Could you check a few things on this model? Use its own coordinates, in mm. A direction names the side the tool comes from. Give positions to 0.01 mm unless a question says otherwise; leave off trailing zeros. Loops run counter-clockwise (first coordinate to the right, second up) from the corner with the lowest first, then second, coordinate; pieces in that order, holes last. Notation, with made-up numbers: (-31, -33.5) -> (17, -33.5) arc R23 ccw to (17, -9.5) -> close; hole circle Ø5 at (-8.5, 16.25). An arc over 180 degrees is marked (long way). Put each result on its own line as item: value.
Autodesk Inventor part; units mm, degrees
ref_plane "bnt_nut_1_XY" through (0, 0, 0) normal (1, 0, 0) x (0, 0, -1)
ref_plane "bnt_nut_1_YZ" through (0, 0, 0) normal (0, 0, -1) x (0, 1, 0)
ref_plane "bnt_nut_1_ZX" through (0, 0, 0) normal (0, 1, 0) x (1, 0, 0)
sketch "Sketch_1" plane through (0, 0, 0) normal (1, 0, 0) x (0, 1, 0)
  line L0 (16.56, 24) -> (9, 24)
  line L1 (9, 24) -> (7.56, 22.56)
  line L2 (7.56, 22.56) -> (-13.14, 22.56)
  line L3 (-13.14, 22.56) -> (-13.14, 18)
  arc A0 (-13.14, 18) -> (-23.4, 9.44) centre (-13.3579, 7.8323) ccw
  line L4 (-23.4, 9.44) -> (-23.4, -9.44)
  arc A1 (-23.4, -9.44) -> (-13.14, -18) centre (-13.3579, -7.8323) ccw
  line L5 (-13.14, -18) -> (-13.14, -22.56)
  line L6 (-13.14, -22.56) -> (7.56, -22.56)
  line L7 (7.56, -22.56) -> (9, -24)
  line L8 (9, -24) -> (16.56, -24)
  line L9 (16.56, -24) -> (18, -22.56)
  line L10 (18, -22.56) -> (18, -9.44)
  line L11 (18, -9.44) -> (16.56, -8)
  line L12 (16.56, -8) -> (16.56, 8)
  line L13 (16.56, 8) -> (18, 9.44)
  line L14 (18, 9.44) -> (18, 22.56)
  line L15 (18, 22.56) -> (16.56, 24)
  circle A2 centre (0, 0) radius 10
extrude "Extrusion1" add sketch "Sketch_1" along normal blind 58
sketch "Sketch_2" plane through (29, 0, 0) normal (0.682, 0, 0.7314) x (0.7314, 0, -0.682)
  line L0 (-29, -24.55) -> (-4.4539, -24.55)
  arc A0 (-4.4539, -24.55) -> (4.4539, -24.55) centre (0, -23.4) ccw
  line L1 (4.4539, -24.55) -> (29, -24.55)
  line L2 (29, -24.55) -> (29, -23.4)
  line L3 (29, -23.4) -> (-29, -23.4)
  line L4 (-29, -23.4) -> (-29, -24.55)
extrude "Extrusion2" add sketch "Sketch_2" along normal mid plane 58
sketch "Sketch_3" plane through (0, -23.4, 0) normal (0, 1, 0) x (1, 0, 0)
  line L0 (-29, -58) -> (87, -58)
  line L1 (87, -58) -> (87, 58)
  line L2 (87, 58) -> (-29, 58)
  line L3 (-29, 58) -> (-29, -58)
  line L4 (9.6667, -9.44) -> (48.3333, -9.44)
  line L5 (48.3333, -9.44) -> (48.3333, 9.44)
  line L6 (48.3333, 9.44) -> (9.6667, 9.44)
  line L7 (9.6667, 9.44) -> (9.6667, -9.44)
extrude "Extrusion3" cut sketch "Sketch_3" against normal blind 4.6
sketch "Sketch_4" plane through (0, 0, 0) normal (0, 0, 1) x (1, 0, 0)
  line L0 (13.4367, -26.15) -> (13.4367, -24.55)
  line L1 (13.4367, -24.55) -> (15.4367, -24.55)
  line L2 (15.4367, -24.55) -> (15.4367, -25.75)
  arc A0 (15.0367, -26.15) -> (15.4367, -25.75) centre (15.0367, -25.75) ccw
  line L3 (15.0367, -26.15) -> (13.4367, -26.15)
  line L4 (13.4367, -26.15) -> (13.4367, -24.55)
revolve "Revolution1" add sketch "Sketch_4" angle 360 about axis through (13.4367, -26.15, 0) along (0, -1, 0)
sketch "Sketch_5" plane through (0, 0, 0) normal (0, 0, 1) x (1, 0, 0)
  line L0 (44.5633, -26.15) -> (44.5633, -24.55)
  line L1 (44.5633, -24.55) -> (46.5633, -24.55)
  line L2 (46.5633, -24.55) -> (46.5633, -25.75)
  arc A0 (46.1633, -26.15) -> (46.5633, -25.75) centre (46.1633, -25.75) ccw
  line L3 (46.1633, -26.15) -> (44.5633, -26.15)
  line L4 (44.5633, -26.15) -> (44.5633, -24.55)
revolve "Revolution2" add sketch "Sketch_5" angle 360 about axis through (44.5633, -26.15, 0) along (0, -1, 0)
sketch "Sketch_6" plane through (0, -26.15, 0) normal (0, 1, 0) x (1, 0, 0)
  line L0 (43.5633, 0.15) -> (43.5633, -0.15)
  line L1 (43.5633, -0.15) -> (44.4133, -0.15)
  line L2 (44.4133, -0.15) -> (44.4133, -1)
  line L3 (44.4133, -1) -> (44.7133, -1)
  line L4 (44.7133, -1) -> (44.7133, -0.15)
  line L5 (44.7133, -0.15) -> (45.5633, -0.15)
  line L6 (45.5633, -0.15) -> (45.5633, 0.15)
  line L7 (45.5633, 0.15) -> (44.7133, 0.15)
  line L8 (44.7133, 0.15) -> (44.7133, 1)
  line L9 (44.7133, 1) -> (44.4133, 1)
  line L10 (44.4133, 1) -> (44.4133, 0.15)
  line L11 (44.4133, 0.15) -> (43.5633, 0.15)
extrude "Extrusion4" cut sketch "Sketch_6" along normal blind 0.8
sketch "Sketch_7" plane through (0, -26.15, 0) normal (0, 1, 0) x (1, 0, 0)
  line L0 (12.4367, 0.15) -> (12.4367, -0.15)
  line L1 (12.4367, -0.15) -> (13.2867, -0.15)
  line L2 (13.2867, -0.15) -> (13.2867, -1)
  line L3 (13.2867, -1) -> (13.5867, -1)
  line L4 (13.5867, -1) -> (13.5867, -0.15)
  line L5 (13.5867, -0.15) -> (14.4367, -0.15)
  line L6 (14.4367, -0.15) -> (14.4367, 0.15)
  line L7 (14.4367, 0.15) -> (13.5867, 0.15)
  line L8 (13.5867, 0.15) -> (13.5867, 1)
  line L9 (13.5867, 1) -> (13.2867, 1)
  line L10 (13.2867, 1) -> (13.2867, 0.15)
  line L11 (13.2867, 0.15) -> (12.4367, 0.15)
extrude "Extrusion5" cut sketch "Sketch_7" along normal blind 0.8
sketch "Sketch8" plane through (0, -13.14, 22.56) normal (0, 0, 1) x (1, 0, 0)
  point P0 (10, 11.14)
hole "Hole1" at (10, -2, 22.56) direction (0, 0, -1) diameter 4.917 depth 14.1406 tip angle 120 countersink diameter 6 countersink angle 90
sketch "Sketch9" plane through (0, 18, -9.44) normal (0, 1, 0) x (1, 0, 0)
  point P0 (11.5, 8.06)
hole "Hole2" at (11.5, 18, -17.5) direction (0, -1, 0) diameter 4.917 depth 13.1406 tip angle 120 countersink diameter 6 countersink angle 90
pattern_linear "Rectangular Pattern1" count 2 spacing 35 along (1, 0, 0) count 2 spacing 35 along (0, 0, 1) of "Hole2"
ref_plane "bnt_nut_1_XY" through (0, 0, 0) normal (1, 0, 0) x (0, 0, -1)
ref_plane "bnt_nut_1_YZ" through (0, 0, 0) normal (0, 0, -1) x (0, 1, 0)
ref_plane "bnt_nut_1_ZX" through (0, 0, 0) normal (0, 1, 0) x (1, 0, 0)
properties part number "BNT 2010-2.6 Nut"
1. I'm going to push flat-ended pins straight in: pin 1 (0.6 mm diameter, centred on x = 44, y = -26, fed in from -Z); pin 2 (1 mm diameter, centred on x = 44.5, z = -0.5, fed in from -Y); pin 3 (3 mm diameter, centred on x = 21, z = 0, fed in from +Y). Where does each tip first touch, or does it pass through?
Recorded:
pin 1: stops at z = -1.97
pin 2: stops at y = -26.15
pin 3: stops at y = 16.56
2. I need wall thicknesses on line 1 (X direction, y = 8.5, z = -17.5); line 2 (Z direction, x = 16.5, y = 0); line 3 (Y direction, x = 15.5, z = 0.5). Which ranges of each line are inside material? Lowest first, please.
Recorded:
line 1: x = 0 to 9.04, 13.96 to 44.04, 48.96 to 58
line 2: z = -22.56 to -10, 10 to 22.56
line 3: y = -24.55 to -9.99, 9.99 to 16.56
3. For faces 1 (the face through (29, 16.56, 0)), 2 (the face through (33, -25, 9.44)), 3 (the face through (46.41, -25.16, -0.77)), which set-ups out of +Z, -Z, +X, -X, +Y, -Y let a thin tool reach every point of the face, with its end or its side?
Recorded:
face 1: +X, -X, +Y
face 2: +Z, +X, -X, -Y
face 3: -Y
4. If we section it at B-B (y = -2): List the corners of the cut face in (x, z) for me, then the cut area to 3 significant figures.
Recorded:
outline: (0, -22.56) -> (58, -22.56) -> (58, -9.8) -> (0, -9.8) -> close; (0, 9.8) -> (7.54, 9.8) -> (7.54, 22.02) -> (7, 22.56) -> (0, 22.56) -> close; (12.46, 9.8) -> (58, 9.8) -> (58, 22.56) -> (13, 22.56) -> (12.46, 22.02) -> close
area: 1,420 mm^2
5. Thinking about a two-plate mould opening in X: for faces 4 (the face through (48, 11.07, -19.45)), 5 (the face through (25, -25, -9.44)), which applies, pulls with the +X half, pulls with the -X half, needs draft (parallel to the pull), parting line crosses it, or undercut?
Recorded:
face 4: undercut
face 5: needs draft
6. If we section it at A-A (y = -9): List the corners of the cut face in (x, z) for me, then the cut area to 3 significant figures.
Recorded:
outline: (0, -22.56) -> (58, -22.56) -> (58, -4.36) -> (0, -4.36) -> close; (0, 4.36) -> (58, 4.36) -> (58, 22.56) -> (0, 22.56) -> close
area: 2,110 mm^2
7. If we section it at C-C (y = -16): List the corners of the cut face in (x, z) for me, then the cut area to 3 significant figures.
Recorded:
outline: (0, -17.65) -> (58, -17.65) -> (58, 17.65) -> (0, 17.65) -> close
area: 2,050 mm^2
